The listing builds one solid part. Answer for the finished solid, in the listing's coordinates (mm). Face numbers are marked on the shaded views. A direction names the side the tool comes from. Give positions to 0.01 mm unless a question says otherwise; leave off trailing zeros. Loops run counter-clockwise (first coordinate to the right, second up) from the corner with the lowest first, then second, coordinate; pieces in that order, holes last. Notation, with made-up numbers: (-21.75, 35) - (-0.75, 35) arc R31 cw to (-0.75, 68) - close; hole circle Ø9 at (-22.75, 68). An arc over 180 degrees is marked (long way). Write each question's results on one line, items separated by ' | '.
from build123d import *

# Parameters (mm, degrees)
F0_R      = 1.7272
F1_DEPTH  = 8.89
F2_W      = 56
F2_H      = 10
F3_DEPTH  = 16.51
F5_DEPTH  = 2.54
F7_DEPTH  = 2.54
F8_R      = 2.0955
F9_DEPTH  = 10.001
F10_R     = 3.556
F11_DEPTH = 4.445


with BuildPart() as f1:
    # F0 (on Front) → F1 (new body)
    with BuildSketch(Plane.XZ):
        Polygon((0, 30), (0, 0), (56, 0), (56, 30), (48, 30), (48, 10), (8, 10), (8, 30), align=None)
        with Locations((4.1, 14.9)):
            Circle(F0_R, mode=Mode.SUBTRACT)
        with Locations((51.9, 14.9)):
            Circle(F0_R, mode=Mode.SUBTRACT)
        with Locations((4.1, 25.1)):
            Circle(F0_R, mode=Mode.SUBTRACT)
        with Locations((51.9, 25.1)):
            Circle(F0_R, mode=Mode.SUBTRACT)
    extrude(amount=F1_DEPTH)

    # F2 (on face) → F3 (join)
    with BuildSketch(Plane.XZ.offset(8.89)):
        with Locations((28, 5)):
            Rectangle(F2_W, F2_H)
    extrude(amount=F3_DEPTH)

    # F4 (on face) → F5 (join)
    with BuildSketch(Plane.YZ.offset(56)):
        with BuildLine():
            Line((0, 30), (-8.89, 30))
            ThreePointArc((-8.89, 30), (-13.550724, 17.032925), (-25.4, 10))
            Line((-25.4, 10), (-25.4, 0))
            Line((-25.4, 0), (0, 0))
            Line((0, 0), (0, 30))
        make_face()
    extrude(amount=F5_DEPTH)

    # F6 (on face) → F7 (join)
    with BuildSketch(Plane(origin=(0, 0, 0), x_dir=(0, -1, 0), z_dir=(-1, 0, 0))):
        Polygon((8.89, 10), (8.89, 30), (0, 30), (0, 0), (25.4, 0), (25.4, 10), align=None)
        with BuildLine():
            ThreePointArc((25.4, 10), (13.550724, 17.032925), (8.89, 30))
            Line((8.89, 30), (8.89, 10))
            Line((8.89, 10), (25.4, 10))
        make_face()
    extrude(amount=F7_DEPTH)

    # F8 (on face) → F9 (cut, through all)
    with BuildSketch(Plane.XY.offset(10)):
        with Locations((12.73, -12.7)):
            Circle(F8_R)
        with Locations((43.27, -12.7)):
            Circle(F8_R)
    extrude(amount=-F9_DEPTH, mode=Mode.SUBTRACT)

    # F10 (on face) → F11 (cut)
    with BuildSketch(Plane.XY.offset(10)):
        with Locations((12.73, -12.7)):
            Circle(F10_R)
        with Locations((43.27, -12.7)):
            Circle(F10_R)
    extrude(amount=-F11_DEPTH, mode=Mode.SUBTRACT)


solid = f1.part
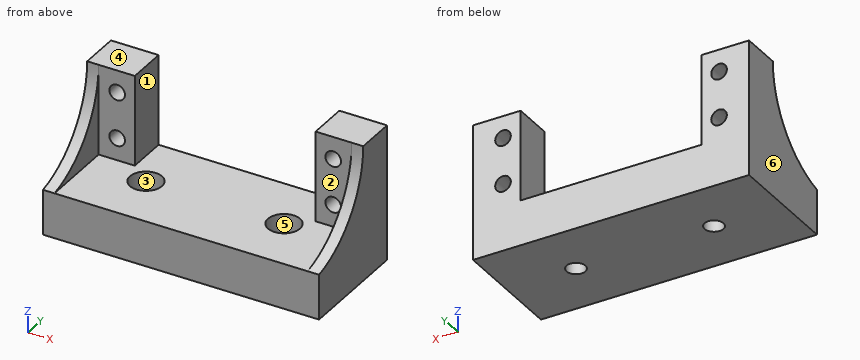
Item 1: A cutting plane is placed at B-B, the plane y = -12.7. Determine the outline of the cut face in (x, z) (1 decimal).
Values found:
outline: (-2.5, 0) - (10.6, 0) - (10.6, 5.6) - (9.2, 5.6) - (9.2, 10) - (0, 10) - (0, 18.1) - (-2.5, 18.1) - close; (14.8, 0) - (41.2, 0) - (41.2, 5.6) - (39.7, 5.6) - (39.7, 10) - (16.3, 10) - (16.3, 5.6) - (14.8, 5.6) - close; (45.4, 0) - (58.5, 0) - (58.5, 18.1) - (56, 18.1) - (56, 10) - (46.8, 10) - (46.8, 5.6) - (45.4, 5.6) - close
Item 2: For the marked faces 1, 2 and 3, determine the directions among +Z, -Z, +X, -X, +Y, -Y from which every point of the face is accessible in a straight line to the end or side of a thin tool.
Values found:
face 1: +Z, +Y, -Y | face 2: +Z, -Y | face 3: +Z
Item 3: A cutting plane is placed at D-D, the plane x = 12.73. Determine the outline of the cut face in (y, z) (1 decimal).
Values found:
outline: (-25.4, 0) - (-14.8, 0) - (-14.8, 5.6) - (-16.3, 5.6) - (-16.3, 10) - (-25.4, 10) - close; (-10.6, 0) - (0, 0) - (0, 10) - (-9.1, 10) - (-9.1, 5.6) - (-10.6, 5.6) - close
Item 4: Flat-ended cylindrical pins translate along their axes: P1, Ø8, axis at x = 13, y = -12, coming from the +Z side; P2, Ø3.5, axis at x = 12.73, y = -12.7, coming from the -Z side; P3, Ø5.5, axis at x = 43.27, y = -12.7, coming from the +Z side (3 decimals); P4, Ø5.5, axis at x = 4.1, z = 14.9, coming from the -Y side. Find the tip coordinate at first contact, or state that the pin passes through.
Values found:
P1: stops at z = 10 | P2: passes through | P3: stops at z = 5.555 | P4: stops at y = -8.89
Item 5: For a pull along X with two mould halves and no side action, classify the marked faces 4, 5 and 6 as released by +X, released by -X, zero draft, split by the parting line, or undercut.
Values found:
face 4: zero draft | face 5: undercut | face 6: released by -X
Item 6: A cutting plane is placed at A-A, the plane x = 51.9. Determine the outline of the cut face in (y, z), plus the area to 3 significant figures.
Values found:
outline: (-25.4, 0) - (0, 0) - (0, 13.17) - (-8.89, 13.17) - (-8.89, 10) - (-25.4, 10) - close; (-8.89, 16.63) - (0, 16.63) - (0, 23.37) - (-8.89, 23.37) - close; (-8.89, 26.83) - (0, 26.83) - (0, 30) - (-8.89, 30) - close | area: 370 mm²
Item 7: A cutting plane is placed at C-C, the plane z = 24.5. Determine the outline of the cut face in (x, y).
Values found:
outline: (-2.54, -9.65) - (0, -9.65) - (0, -8.89) - (2.48, -8.89) - (2.48, 0) - (-2.54, 0) - close; (5.72, -8.89) - (8, -8.89) - (8, 0) - (5.72, 0) - close; (48, -8.89) - (50.28, -8.89) - (50.28, 0) - (48, 0) - close; (53.52, -8.89) - (56, -8.89) - (56, -9.65) - (58.54, -9.65) - (58.54, 0) - (53.52, 0) - close
Item 8: Find the intervals of material crossed by line 1 along X through (y, z) = (-6, 15); line 2 along Z through (x, y) = (51.9, -4.5); line 3 along X through (y, z) = (-2.5, 18), in increasing order. Write a range as [from, to].
Values found:
line 1: x = [-2.54, 2.38], [5.82, 8], [48, 50.18], [53.62, 58.54] | line 2: z = [0, 13.17], [16.63, 23.37], [26.83, 30] | line 3: x = [-2.54, 8], [48, 58.54]
